Verification items for the finished model (mm, model axes). A direction names the side the tool comes from. Round coordinates to 2 decimals unless told otherwise and drop trailing zeros. Loops run counter-clockwise (first coordinate to the right, second up) from the corner with the lowest first, then second, coordinate; pieces in that order, holes last.
from build123d import *

# Parameters (mm, degrees)
F0_R      = 101.6404719392
F1_DEPTH  = 6.35
F2_R      = 12.7
F3_R      = 12.7
F4_R      = 12.7
F5_R      = 12.7
F6_R      = 12.8569190272
F7_DEPTH  = 6.35
F9_D      = 12.5984
F9_DEPTH  = 4.7498
F9_TIP    = 3.7849412114
F11_D     = 12.5984
F11_DEPTH = 4.7498
F11_TIP   = 3.7849412114
F12_D     = 10.0584


with BuildPart() as f1:
    # F0 (on Top) → F1 (new body)
    with BuildSketch(Plane.XY):
        Circle(F0_R)
        with BuildLine():
            ThreePointArc((91.2431268086, 12.6268099993), (91.8950293011, 6.328357632), (92.112672964, 0))
            ThreePointArc((92.112672964, 0), (69.5117488598, -60.438905442), (12.7997798845, -91.2190229912))
            ThreePointArc((12.7997798845, -91.2190229912), (6.4154691053, -91.8889888764), (0, -92.112672964))
            ThreePointArc((0, -92.112672964), (-60.3729648841, -69.5690278189), (-91.194584597, -12.972750701))
            ThreePointArc((-91.194584597, -12.972750701), (-91.8828642012, -6.5025984614), (-92.112672964, 0))
            ThreePointArc((-92.112672964, 0), (-69.5117488598, 60.438905442), (-12.7997798845, 91.2190229912))
            ThreePointArc((-12.7997798845, 91.2190229912), (-6.4154691053, 91.8889888764), (0, 92.112672964))
            ThreePointArc((0, 92.112672964), (60.5047737808, 69.4544229715), (91.2431268086, 12.6268099993))
        make_face(mode=Mode.SUBTRACT)
        with BuildLine():
            Line((19.1497798845, 0), (92.112672964, 0))
            ThreePointArc((92.112672964, 0), (91.8950293011, 6.328357632), (91.2431268086, 12.6268099993))
            Line((91.2431268086, 12.6268099993), (6.35, 12.6268099993))
            ThreePointArc((6.35, 12.6268099993), (1.8598719395, 14.4866819388), (0, 18.9768099993))
            Line((0, 18.9768099993), (0, 92.112672964))
            ThreePointArc((0, 92.112672964), (-6.4154691053, 91.8889888764), (-12.7997798845, 91.2190229912))
            Line((-12.7997798845, 91.2190229912), (-12.7997798845, 6.35))
            ThreePointArc((-12.7997798845, 6.35), (-14.659651824, 1.8598719395), (-19.1497798845, 0))
            Line((-19.1497798845, 0), (-92.112672964, 0))
            ThreePointArc((-92.112672964, 0), (-91.8828642012, -6.5025984614), (-91.194584597, -12.972750701))
            Line((-91.194584597, -12.972750701), (-6.35, -12.972750701))
            ThreePointArc((-6.35, -12.972750701), (-1.8598719395, -14.8326226405), (0, -19.322750701))
            Line((0, -19.322750701), (0, -92.112672964))
            ThreePointArc((0, -92.112672964), (6.4154691053, -91.8889888764), (12.7997798845, -91.2190229912))
            Line((12.7997798845, -91.2190229912), (12.7997798845, -6.35))
            ThreePointArc((12.7997798845, -6.35), (14.659651824, -1.8598719395), (19.1497798845, 0))
        make_face()
    extrude(amount=F1_DEPTH)

    # F2
    f2_edges = [f1.edges().sort_by_distance(p)[0] for p in [
        (-91.194585, -12.972751, 3.175),
        (0, 92.112673, 3.175),
    ]]
    fillet(f2_edges, radius=F2_R)

    # F3
    f3_edges = [f1.edges().sort_by_distance(p)[0] for p in [
        (12.79978, -91.219023, 3.175),
        (-92.112673, 0, 3.175),
    ]]
    fillet(f3_edges, radius=F3_R)

    # F4
    f4_edges = [f1.edges().sort_by_distance(p)[0] for p in [
        (-12.79978, 91.219023, 3.175),
        (92.112673, 0, 3.175),
    ]]
    fillet(f4_edges, radius=F4_R)

    # F5
    f5_edges = [f1.edges().sort_by_distance(p)[0] for p in [
        (91.243127, 12.62681, 3.175),
        (0, -92.112673, 3.175),
    ]]
    fillet(f5_edges, radius=F5_R)

    # F6 (on face) → F7 (join)
    with BuildSketch(Plane.XY.offset(6.35)):
        Circle(F6_R)
    extrude(amount=F7_DEPTH)

    # F9
    with Locations(Plane.XY.offset(12.7)):
        with Locations((0, 0)):
            Hole(F9_D / 2, depth=F9_DEPTH)
            with Locations((0, 0, -(F9_DEPTH + F9_TIP / 2))):  # 118° drill point
                Cone(0, F9_D / 2, F9_TIP, mode=Mode.SUBTRACT)

    # F11
    with Locations(Plane(origin=(0, 0, 0), x_dir=(1, 0, 0), z_dir=(0, 0, -1))):
        with Locations((0, 0)):
            Hole(F11_D / 2, depth=F11_DEPTH)
            with Locations((0, 0, -(F11_DEPTH + F11_TIP / 2))):  # 118° drill point
                Cone(0, F11_D / 2, F11_TIP, mode=Mode.SUBTRACT)

    # F12 (through all)
    with Locations(Plane(origin=(0, 0, 0), x_dir=(1, 0, 0), z_dir=(0, 0, -1))):
        with Locations((0, 0)):
            Hole(F12_D / 2)


solid = f1.part
1. Gauge pin test, flat ends, axial feed: P1, Ø7, axis at y = 39.5, z = 2, coming from the +X side; P2, Ø7, axis at y = 47.5, z = 4, coming from the -X side; P3, Ø7, axis at y = -35, z = 4, coming from the +X side. Record the tip position at first contact, or that the pin passes through.
2. Tool access check on faces 1 (the face through (-2.79, -12.55, 9.48)), 2 (the face through (5, 3.83, 2.41)), 3 (the face through (41, 12.627, 3)), 4 (the face through (6, 3, 12.7)). Record the directions out of +Z, -Z, +X, -X, +Y, -Y that give a thin tool (end or side, any length) a straight path to the whole face; none if there is none.
3. Scan lines: L1, parallel to X at y = -54, z = 1.25; L2, parallel to X at y = 53, z = 5.5; L3, parallel to Y at x = -50.5, z = 2. Record each from-to range of solid material in increasing order.
4. Section check A-A (x = 82). Enter the section's corners in (y, z).
5. Release check for a two-part mould opening along X. For faces 5 (the face through (0, 8, 0)), 6 (the face through (-80.658, -61.847, 3.131)), 7 (the face through (59.045, 70.7, 3.131)) record: released by +X, released by -X, zero draft, split by the parting line, or undercut.
6. Section check B-B (y = 27). Enter the section's corners in (x, z) (3 decimals).
Taken from the geometry:
1. P1: stops at x = 95.05
1. P2: stops at x = -91.62
1. P3: stops at x = 96.64
2. face 1: +Z
2. face 2: -Z
2. face 3: +Z, -Z
2. face 4: +Z, +X, -X, +Y, -Y
3. L1: x = -86.11 to -74.62, 0 to 12.8, 74.62 to 86.11
3. L2: x = -86.73 to -75.34, -12.8 to 0, 75.34 to 86.73
3. L3: y = -88.21 to -77.04, -12.97 to 0, 77.04 to 88.21
4. outline: (-60.06, 0) - (-41.96, 0) - (-41.96, 6.35) - (-60.06, 6.35) - close; (-0.52, 0) - (14.56, 0) - (14.56, 6.35) - (-0.52, 6.35) - close; (41.96, 0) - (60.06, 0) - (60.06, 6.35) - (41.96, 6.35) - close
5. face 5: zero draft
5. face 6: split by the parting line
5. face 7: undercut
6. outline: (-97.989, 0) - (-88.067, 0) - (-88.067, 6.35) - (-97.989, 6.35) - close; (-12.8, 0) - (0, 0) - (0, 6.35) - (-12.8, 6.35) - close; (87.855, 0) - (97.989, 0) - (97.989, 6.35) - (87.855, 6.35) - close
